Design review of the part shown in the three views and the two pictorial views. Dimensions are in mm from the part's minimum x, y and z. A direction names the side the tool comes from. Coordinates: 2 decimals unless noted, no trailing zeros. Write each loop counter-clockwise with the first axis right and the second up, starting at its lowest first coordinate (ties: lowest second). Pieces come first, ordered by that corner, then holes. Notation, with made-up numbers: M -39,66.25 L -12,66.25 A37 ccw -12,103.25 Z; hole C -30,71 d7. An arc over 180 degrees is marked long. One line per question, with ' | ' between items.
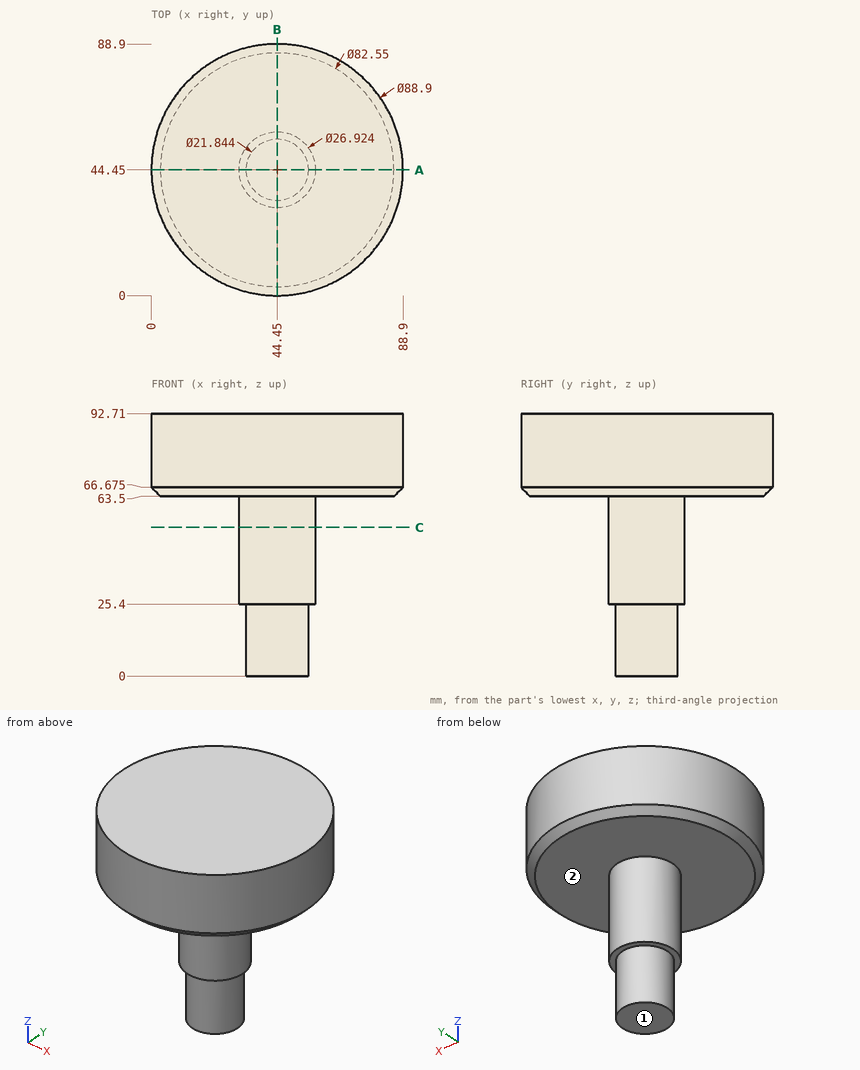
1. For line 1 along Z through (x, y) = (64.5, 48); line 2 along Y through (x, z) = (47.5, 69); line 3 along Z through (x, y) = (55, 51), list the stretches that pass through material, from the lowest coordinate up.
Computed values:
line 1: z = 63.5 to 92.71 | line 2: y = 0.1 to 88.8 | line 3: z = 25.4 to 92.71
2. Clearance check with flat-ended pins moving along their axes: P1, Ø3, axis at x = 26, y = 42, coming from the -Z side; P2, Ø10, axis at x = 27.5, z = 54.5, coming from the +Y side; P3, Ø1.5, axis at x = 17, z = 69.5, coming from the +Y side. State where each tip first meets the part, or that it passes through.
Computed values:
P1: stops at z = 63.5 | P2: stops at y = 50.65 | P3: stops at y = 79.99
3. Take a section at A-A on y = 44.45. State the section outline as (x, z) points (3 decimals).
Computed values:
outline: M 0,66.675 L 3.175,63.5 L 30.988,63.5 L 30.988,25.4 L 33.528,25.4 L 33.528,0 L 55.372,0 L 55.372,25.4 L 57.912,25.4 L 57.912,63.5 L 85.725,63.5 L 88.9,66.675 L 88.9,92.71 L 0,92.71 Z
4. Take a section at C-C on z = 52.5. State the section outline as (x, y) points, plus the area to 3 significant figures.
Computed values:
outline: C 44.45,44.45 d26.92 | area: 569 mm2
5. Machinability: for the marked faces 1 and 2, which of the approach directions +Z, -Z, +X, -X, +Y, -Y give a long, thin tool a straight path to every point of the face, cutting with its end or side? Answer none if there is none.
Computed values:
face 1: -Z, +X, -X, +Y, -Y | face 2: -Z
